from build123d import *

# Parameters (mm, degrees)
CYLINDER001_R     = 5.5
CYLINDER001_DEPTH = 10
BOX001_W          = 60
BOX001_H          = 60
BOX001_DEPTH      = 60
PAD_DEPTH         = 2
PAD001_DEPTH      = 2
CYLINDER_R        = 7
CYLINDER_DEPTH    = 10
SKETCH_R          = 5.5
POCKET_DEPTH      = 10.001
BOX_W             = 30
BOX_H             = 30
BOX_DEPTH         = 2
SKETCH001_R       = 1.6
POCKET001_DEPTH   = 2.001


with BuildPart() as cylinder001:
    # Cylinder001 → Cylinder001 (new body)
    with BuildSketch(Plane.XY):
        Circle(CYLINDER001_R)
    extrude(amount=CYLINDER001_DEPTH)


with BuildPart() as cube001:
    # Box001 → Box001 (new body)
    with BuildSketch(Plane(origin=(-30, -30, 10), x_dir=(1, 0, 0), z_dir=(0, 0, 1))):
        with Locations((30, 30)):
            Rectangle(BOX001_W, BOX001_H)
    extrude(amount=BOX001_DEPTH)


with BuildPart() as pad:
    # Sketch002 → Pad (new body)
    with BuildSketch(Plane.XZ.offset(-1)):
        Polygon((-15, 0), (0, 18), (15, 0), align=None)
    extrude(amount=PAD_DEPTH)


with BuildPart() as pad001:
    # Sketch003 → Pad001 (new body)
    with BuildSketch(Plane.YZ.offset(-1)):
        Polygon((-15, 0), (0, 18), (15, 0), align=None)
    extrude(amount=PAD001_DEPTH)


with BuildPart() as pocket:
    # Cylinder → Cylinder (new body)
    with BuildSketch(Plane.XY):
        Circle(CYLINDER_R)
    extrude(amount=CYLINDER_DEPTH)

    # Sketch → Pocket (cut, through all)
    with BuildSketch(Plane.XY.offset(10)):
        Circle(SKETCH_R)
    extrude(amount=-POCKET_DEPTH, mode=Mode.SUBTRACT)


with BuildPart() as cut001:
    # Box → Box (new body)
    with BuildSketch(Plane(origin=(-15, -15, 0), x_dir=(1, 0, 0), z_dir=(0, 0, 1))):
        with Locations((15, 15)):
            Rectangle(BOX_W, BOX_H)
    extrude(amount=BOX_DEPTH)

    # Sketch001 → Pocket001 (cut, through all)
    with BuildSketch(Plane(origin=(-15, -15, 2), x_dir=(1, 0, 0), z_dir=(0, 0, 1))):
        with Locations((4, 4)):
            Circle(SKETCH001_R)
        with Locations((26, 26)):
            Circle(SKETCH001_R)
        with Locations((26, 4)):
            Circle(SKETCH001_R)
        with Locations((4, 26)):
            Circle(SKETCH001_R)
    extrude(amount=-POCKET001_DEPTH, mode=Mode.SUBTRACT)

    # Fusion: union Pad, Pad001, Pocket
    add(pad.part)
    add(pad001.part)
    add(pocket.part)

    # Cut: cut Cube001
    add(cube001.part, mode=Mode.SUBTRACT)

    # Cut001: cut Cylinder001
    add(cylinder001.part, mode=Mode.SUBTRACT)


solid = cut001.part
Source: CAD feature listing. Evaluate the final solid. Frame: model axes, mm. A direction names the side the tool comes from. Give positions to 0.01 mm unless a question says otherwise; leave off trailing zeros. Write each loop counter-clockwise with the first axis right and the second up, starting at its lowest first coordinate (ties: lowest second). Pieces come first, ordered by that corner, then holes. Notation, with made-up numbers: M 67.25,38 L 84.25,38 A35 ccw 84.25,70 Z; hole C -15.75,34 d11. An arc over 180 degrees is marked long. Return JSON: item names as keys, results as strings. Group by question number.
1) Cut plane B-B, the plane y = 0. Output: boundary loops of the cut face in (x, z), plus the area to 3 significant figures.
2) Cut plane D-D, the plane x = -11.25. Output: boundary loops of the cut face in (y, z), plus the area to 3 significant figures.
3) Material intervals for line 1 along Y through (x, z) = (11, 1.45); line 2 along Z through (x, y) = (12, -4.5); line 3 along X through (y, z) = (-7.5, 6.5), sorted ascending. Write a range as [from, to].
4) Cut plane A-A, the plane y = -11. Output: boundary loops of the cut face in (x, z).
5) Pin query (flat end, axial travel): P1, Ø5, axis at x = 11, z = 7.5, coming from the -Y side; P2, Ø1.9, axis at y = 9, z = 6.5, coming from the +X side; P3, Ø5, axis at x = -1.5, z = 7.5, coming from the -Y side. Return the tip coordinate at first contact, or that it passes through.
6) Set-up query: faces 4 (the face through (-9, -1, 4)), 5 (the face through (-1, 9, 4)), 6 (the face through (1, 9, 4)). Return all of +Z, -Z, +X, -X, +Y, -Y with unobstructed straight access to the full face (end or side cutting, diameter ignored); none if empty.
7) Pull-direction query (Y, two-part tool) for faces 1 (the face through (0, -15, 1)), 2 (the face through (1, -9, 4)), 3 (the face through (-12.6, -10.93, 1.01)); classes: pulls with the +Y half, pulls with the -Y half, needs draft (parallel to the pull), parting line crosses it, or undercut.
8) Cut plane C-C, the plane z = 3. Output: boundary loops of the cut face in (x, y), plus the area to 3 significant figures.
Recorded:
{
 "1": {"outline": "M -15,0 L -5.5,0 L -5.5,10 L -7,10 L -7,9.6 L -13.33,2 L -15,2 Z; M 5.5,0 L 15,0 L 15,2 L 13.33,2 L 7,9.6 L 7,10 L 5.5,10 Z", "area": "110 mm²"},
 "2": {"outline": "M -15,0 L -12.58,0 L -12.58,2 L -15,2 Z; M -9.42,0 L 9.42,0 L 9.42,2 L 1,2 L 1,4.5 L -1,4.5 L -1,2 L -9.42,2 Z; M 12.58,0 L 15,0 L 15,2 L 12.58,2 Z", "area": "52.4 mm²"},
 "3": {"line 1": "y = [-15, -12.6], [-9.4, 9.4], [12.6, 15]", "line 2": "z = [0, 2]", "line 3": "x = [-1, 1]"},
 "4": {"outline": "M -15,0 L -12.6,0 L -12.6,2 L -15,2 Z; M -9.4,0 L 9.4,0 L 9.4,2 L 1,2 L 1,4.8 L -1,4.8 L -1,2 L -9.4,2 Z; M 12.6,0 L 15,0 L 15,2 L 12.6,2 Z"},
 "5": {"P1": "stops at y = -1", "P2": "stops at x = 1", "P3": "stops at y = -10.79"},
 "6": {"face 4": "+Z, -X, -Y", "face 5": "+Z, -X, +Y", "face 6": "+Z, +X, +Y"},
 "7": {"face 1": "pulls with the -Y half", "face 2": "needs draft", "face 3": "undercut"},
 "8": {"outline": "M -12.5,-1 L -6.93,-1 A7 ccw -1,-6.93 L -1,-12.5 L 1,-12.5 L 1,-6.93 A7 ccw 6.93,-1 L 12.5,-1 L 12.5,1 L 6.93,1 A7 ccw 1,6.93 L 1,12.5 L -1,12.5 L -1,6.93 A7 ccw -6.93,1 L -12.5,1 Z; hole C 0,0 d11", "area": "103 mm²"}
}
